Build history of the part. All positions in model axes, mm. A direction names the side the tool comes from. Give positions to 0.01 mm unless a question says otherwise; leave off trailing zeros. Loops run counter-clockwise (first coordinate to the right, second up) from the corner with the lowest first, then second, coordinate; pieces in that order, holes last. Notation, with made-up numbers: (-12.75, -21) -> (19.25, -21) arc R13 cw to (19.25, -14) -> close; hole circle Ø8 at (87.25, -1.75). An arc over 180 degrees is marked (long way). One line per question, with ' | ' between items. Start each with the question number.
(1) 3-axis set-ups, long thin cutter, end or side, ignore diameter. For faces 4 (the face through (-19.05, 3, 70)), 5 (the face through (34.925, 3, -24)), 6 (the face through (-25, 2.54, 21)), 7 (the face through (-70, 3, -19.05)), 8 (the face through (19.05, 3, 71)): which of +Z, -Z, +X, -X, +Y, -Y reach the whole face in a straight line?
(2) Drill centre lines: L1, parallel to Z at x = -23, y = 2.5 (3 decimals); L2, parallel to X at y = 4.5, z = 19 (1 decimal); L3, parallel to X at y = 5, z = -17 (1 decimal). Where is each one in solid material? Low to high. Write a range as from..to.
(3) Flat gauge pins, fed straight in: pin 1 Ø1.9 at (x, y) = (72.5, 3) entering from +Z; pin 2 Ø3.5 at (x, z) = (15.875, 98.425) entering from -Y; pin 3 Ø3 at (y, z) = (4.5, -24.5) entering from +X (3 decimals); pin 4 Ø1.9 at (x, y) = (-25, 2) entering from +Z (3 decimals). Where does each tip first touch, or does it go through?
(4) Slice it at D-D, the plane y = 1.5. Give the number of separate pieces and of enclosed holes in the cut face, then the cut area to 3 significant figures.
(5) Slice it at B-B, the plane x = -72.5. Write the cut outline in (y, z).
(6) Mould opens along X. For faces 1 (the face through (-33.11, 3.13, 33.02)), 2 (the face through (34.925, 3, 24)), 3 (the face through (-0.05, 3.13, 14.96)) say: pulls with the +X half, pulls with the -X half, needs draft (parallel to the pull), parting line crosses it, or undercut.
(7) Slice it at C-C, the plane z = 68. Write the cut outline in (x, y).
```python
from build123d import *

# Parameters (mm, degrees)
BOSS_EXTRU_1_DEPTH           = 6.35
ENL_V_MAT_EXTRU_1_REACH      = 152.112
ESQUISSE2_R                  = 2.1844
ENL_V_MAT_EXTRU_2_DEPTH      = 2.54
ENL_V_MAT_EXTRU_3_REACH      = 152.112
ESQUISSE5_R                  = 1.89865
ENL_V_MAT_EXTRU_4_DEPTH      = 151.112071772
R_P_TITION_CIRCULAIRE1_COUNT = 4


with BuildPart() as part:
    # Esquisse1 → Boss.-Extru.1 (new body)
    with BuildSketch(Plane(origin=(0, 0, 0), x_dir=(1, 0, 0), z_dir=(0, 1, 0))):
        with BuildLine():
            Line((19.049999994, 106.045), (-19.050000006, 106.045))
            Line((-19.050000006, 106.045), (-19.050000006, 34.925))
            Line((-19.050000006, 34.925), (-28.575, 34.925))
            ThreePointArc((-28.575, 34.925), (-33.065128061, 33.065128061), (-34.925, 28.575))
            Line((-34.925, 28.575), (-34.925, 19.05))
            Line((-34.925, 19.05), (-106.045, 19.05))
            Line((-106.045, 19.05), (-106.045, -19.05))
            Line((-106.045, -19.05), (-34.925, -19.05))
            Line((-34.925, -19.05), (-34.925, -28.575))
            ThreePointArc((-34.925, -28.575), (-33.065128061, -33.065128061), (-28.575, -34.925))
            Line((-28.575, -34.925), (-19.05, -34.925))
            Line((-19.05, -34.925), (-19.05, -106.045))
            Line((-19.05, -106.045), (19.05, -106.045))
            Line((19.05, -106.045), (19.05, -34.925))
            Line((19.05, -34.925), (28.575, -34.925))
            ThreePointArc((28.575, -34.925), (33.065128061, -33.065128061), (34.925, -28.575))
            Line((34.925, -28.575), (34.925, -19.05))
            Line((34.925, -19.05), (106.055502293, -19.05))
            Line((106.055502293, -19.05), (106.055502293, 19.05))
            Line((106.055502293, 19.05), (34.925, 19.05))
            Line((34.925, 19.05), (34.925, 28.575))
            ThreePointArc((34.925, 28.575), (33.065128061, 33.065128061), (28.575, 34.925))
            Line((28.575, 34.925), (19.049999994, 34.925))
            Line((19.049999994, 34.925), (19.049999994, 106.045))
        make_face()
    extrude(amount=BOSS_EXTRU_1_DEPTH)

    # Esquisse2 → Enlèv. mat.-Extru.1 (cut, up to next)
    with BuildSketch(Plane.XZ, mode=Mode.PRIVATE) as enl_v_mat_extru_1_sk1:
        with Locations(Location((-20.474983956, 27.659188853, 0), (0, 0, 270))):
            Circle(ESQUISSE2_R)
    enl_v_mat_extru_1_tool1 = extrude(enl_v_mat_extru_1_sk1.sketch, amount=-ENL_V_MAT_EXTRU_1_REACH, mode=Mode.PRIVATE) & part.part
    # Esquisse2 → Enlèv. mat.-Extru.1 (cut, up to next)
    with BuildSketch(Plane.XZ, mode=Mode.PRIVATE) as enl_v_mat_extru_1_sk2:
        with Locations(Location((-27.659188853, 20.474983956, 0), (0, 0, 270))):
            Circle(ESQUISSE2_R)
    enl_v_mat_extru_1_tool2 = extrude(enl_v_mat_extru_1_sk2.sketch, amount=-ENL_V_MAT_EXTRU_1_REACH, mode=Mode.PRIVATE) & part.part
    # Esquisse2 → Enlèv. mat.-Extru.1 (cut, up to next)
    with BuildSketch(Plane.XZ, mode=Mode.PRIVATE) as enl_v_mat_extru_1_sk3:
        with Locations(Location((13.111173937, -5.92696904, 0), (0, 0, 270))):
            Circle(ESQUISSE2_R)
    enl_v_mat_extru_1_tool3 = extrude(enl_v_mat_extru_1_sk3.sketch, amount=-ENL_V_MAT_EXTRU_1_REACH, mode=Mode.PRIVATE) & part.part
    # Esquisse2 → Enlèv. mat.-Extru.1 (cut, up to next)
    with BuildSketch(Plane.XZ, mode=Mode.PRIVATE) as enl_v_mat_extru_1_sk4:
        with Locations(Location((5.92696904, -13.111173937, 0), (0, 0, 270))):
            Circle(ESQUISSE2_R)
    enl_v_mat_extru_1_tool4 = extrude(enl_v_mat_extru_1_sk4.sketch, amount=-ENL_V_MAT_EXTRU_1_REACH, mode=Mode.PRIVATE) & part.part
    add(enl_v_mat_extru_1_tool1.solids().sort_by_distance((-20.474984, 0, 27.659189))[0], mode=Mode.SUBTRACT)
    add(enl_v_mat_extru_1_tool2.solids().sort_by_distance((-27.659189, 0, 20.474984))[0], mode=Mode.SUBTRACT)
    add(enl_v_mat_extru_1_tool3.solids().sort_by_distance((13.111174, 0, -5.926969))[0], mode=Mode.SUBTRACT)
    add(enl_v_mat_extru_1_tool4.solids().sort_by_distance((5.926969, 0, -13.111174))[0], mode=Mode.SUBTRACT)

    # Esquisse3 → Enlèv. mat.-Extru.2 (cut)
    with BuildSketch(Plane.XZ):
        Polygon((16.652426289, -6.875844748), (15.703550581, -3.334592395), (12.162298229, -2.385716687), (9.569921584, -4.978093332), (10.518797292, -8.519345684), (14.060049645, -9.468221392), align=None)
        Polygon((9.468221392, -14.060049645), (8.519345684, -10.518797292), (4.978093332, -9.569921584), (2.385716687, -12.162298229), (3.334592395, -15.703550581), (6.875844748, -16.652426289), align=None)
        Polygon((-17.882607312, 30.251565497), (-21.423859664, 31.200441205), (-24.016236309, 28.608064561), (-23.0673606, 25.066812208), (-19.526108248, 24.1179365), (-16.933731604, 26.710313145), align=None)
        Polygon((-28.608064561, 24.016236309), (-31.200441205, 21.423859664), (-30.251565497, 17.882607312), (-26.710313145, 16.933731604), (-24.1179365, 19.526108248), (-25.066812208, 23.0673606), align=None)
    extrude(amount=-ENL_V_MAT_EXTRU_2_DEPTH, mode=Mode.SUBTRACT)

    # Esquisse4 → Enlèv. mat.-Extru.3 (cut, up to next)
    with BuildSketch(Plane.XZ, mode=Mode.PRIVATE) as enl_v_mat_extru_3_sk1:
        Polygon((-29.419319053, 14.512093892), (-14.512093892, 29.419319053), (14.8174226, 0.089802561), (-0.089802561, -14.8174226), align=None)
    enl_v_mat_extru_3_tool1 = extrude(enl_v_mat_extru_3_sk1.sketch, amount=-ENL_V_MAT_EXTRU_3_REACH, mode=Mode.PRIVATE) & part.part
    add(enl_v_mat_extru_3_tool1.solids().sort_by_distance((-7.300948, 0, 7.300948))[0], mode=Mode.SUBTRACT)

    # Esquisse5 → Enlèv. mat.-Extru.4 (cut, through all)
    with BuildSketch(Plane(origin=(0, 6.35, 0), x_dir=(1, 0, 0), z_dir=(0, 1, 0))):
        with Locations(Location((15.875, -98.425, 0), (0, 0, 270))):
            Circle(ESQUISSE5_R)
        with Locations(Location((-15.875, -98.425, 0), (0, 0, 270))):
            Circle(ESQUISSE5_R)
    enl_v_mat_extru_4 = extrude(amount=-ENL_V_MAT_EXTRU_4_DEPTH, mode=Mode.SUBTRACT)

    # Répétition circulaire1: Enlèv. mat.-Extru.4 ×4 about axis
    r_p_tition_circulaire1_axis = Axis((0, 0, 0), (0, 1, 0))
    for i in range(1, R_P_TITION_CIRCULAIRE1_COUNT):
        add(enl_v_mat_extru_4.rotate(r_p_tition_circulaire1_axis, i * 360 / R_P_TITION_CIRCULAIRE1_COUNT), mode=Mode.SUBTRACT)


solid = part.part
```
Final values:
1) face 4: +Z, -X, +Y, -Y | face 5: -Z, +X, +Y, -Y | face 6: -Y | face 7: -Z, -X, +Y, -Y | face 8: +Z, +X, +Y, -Y
2) L1: -34.925..8.093, 20.931..25.049, 29.624..34.925 | L2: -106..-29.3, -26..-24.9, -4.1..106.1 | L3: -106..-100, -96.9..96.9, 100..106.1
3) pin 1: z = 19.05 | pin 2: through | pin 3: x = 34.925 | pin 4: z = 34.925
4) separate pieces: 1 | enclosed holes: 9 | area: 14,600 mm2
5) outline: (0, -19.05) -> (6.35, -19.05) -> (6.35, 19.05) -> (0, 19.05) -> close
6) face 1: pulls with the -X half | face 2: pulls with the +X half | face 3: undercut
7) outline: (-19.05, 0) -> (19.05, 0) -> (19.05, 6.35) -> (-19.05, 6.35) -> close
